Design review of the part built by this model. Coordinates are the model's own, in mm. A direction names the side the tool comes from. Coordinates: 2 decimals unless noted, no trailing zeros. Write each loop counter-clockwise with the first axis right and the second up, starting at its lowest first coordinate (ties: lowest second). Pieces come first, ordered by that corner, then holes.
Q1. For probe 1 along Y at (x, z) = (13, -22); probe 2 along Y at (x, z) = (19, -21); probe 3 along Z at (x, y) = (21, -9.25), list the stretches that pass through material, from the lowest coordinate up.
Q2. Insertion check: pin 1 (17 mm diameter, centred on x = 12, z = 0.5, fed in from -Y); pin 2 (2 mm diameter, centred on x = 22, y = -1, fed in from -Z); pin 3 (5 mm diameter, centred on y = 0, z = 21, fed in from +X); pin 4 (6.5 mm diameter, centred on y = 1.5, z = 29, fed in from -X). Each pin has a flat end and moves straight along its axis. Give the tip position at first contact, or say it passes through.
Q3. Take a section at A-A (x = 19.5). Give the boundary of the cut face in (y, z).
Q4. Take a section at C-C (y = 3). Give the boundary of the cut face in (x, z).
Q5. Take a section at B-B (x = 31). Give the boundary of the cut face in (y, z) (3 decimals).
Q6. Machinability: for faces 4 (the cylindrical face through (27.34, 11.01, -1.82)), 5 (the flat face through (10.364, 0, 27)), 6 (the flat face through (28, 6, 0)), which of the approach directions +Z, -Z, +X, -X, +Y, -Y give a long, thin tool a straight path to every point of the face, cutting with its end or side? Answer none if there is none.
Q7. Mouldability with a two-part tool opening along Y and no side actions: class faces 1 (the cylindrical face through (25.25, -8.03, -2.76)), 2 (the flat face through (24, 12, -2)), 3 (the cylindrical face through (32.84, 0.08, 4.7)) as pulls with the +Y half, pulls with the -Y half, needs draft (parallel to the pull), parting line crosses it, or undercut.
Q8. Take a section at D-D (z = 15.5). Give the boundary of the cut face in (x, y), and give its area (3 significant figures).
```python
from build123d import *

# Parameters (mm, degrees)
F0_R     = 2
F1_DEPTH = 6
F2_DEPTH = 12
F4_DEPTH = 2
F6_DEPTH = 2


with BuildPart() as f1:
    # F0 (on Front) → F1 (new body, symmetric)
    with BuildSketch(Plane.XZ):
        with BuildLine():
            Line((24.215026, 28.858344), (10.364281, 33.899603))
            Line((10.364281, 33.899603), (10.364281, 25.364181))
            ThreePointArc((10.364281, 25.364181), (27.303004, -2.303471), (5.968233, -26.742105))
            Line((5.968233, -26.742105), (5.968233, -35.4))
            Line((5.968233, -35.4), (12.884546, -35.4))
            Line((12.884546, -35.4), (32.624816, -18.835947))
            Line((32.624816, -18.835947), (37.099572, 6.541656))
            Line((37.099572, 6.541656), (24.215026, 28.858344))
        make_face()
        with Locations((10.764081, -29.574071)):
            Circle(F0_R, mode=Mode.SUBTRACT)
        with Locations((27.255351, -15.735884)):
            Circle(F0_R, mode=Mode.SUBTRACT)
        with Locations((20.229663, 24.108774)):
            Circle(F0_R, mode=Mode.SUBTRACT)
        with Locations((30.993642, 5.465015)):
            Circle(F0_R, mode=Mode.SUBTRACT)
        with BuildLine():
            ThreePointArc((5.968233, -26.742105), (27.303004, -2.303471), (10.364281, 25.364181))
            Line((10.364281, 25.364181), (10.364281, 23.189258))
            ThreePointArc((10.364281, 23.189258), (25.293606, -2.322395), (5.968233, -24.688868))
            Line((5.968233, -24.688868), (5.968233, -26.742105))
        make_face()
    extrude(amount=F1_DEPTH, both=True)

    # F0 (on Front) → F2 (join, symmetric)
    with BuildSketch(Plane.XZ):
        with BuildLine():
            ThreePointArc((5.968233, -24.688868), (25.293606, -2.322395), (10.364281, 23.189258))
            Line((10.364281, 23.189258), (10.364281, 21.189258))
            ThreePointArc((10.364281, 21.189258), (23.471393, -2.344502), (5.968233, -22.820674))
            Line((5.968233, -22.820674), (5.968233, -24.688868))
        make_face()
    extrude(amount=F2_DEPTH, both=True)

    # F3 (on face) → F4 (join)
    with BuildSketch(Plane.XZ.offset(12)):
        with BuildLine():
            Line((5.968233, -24.688868), (5.968233, -26.742105))
            ThreePointArc((5.968233, -26.742105), (27.303004, -2.303471), (10.364281, 25.364181))
            Line((10.364281, 25.364181), (10.364281, 23.189258))
            ThreePointArc((10.364281, 23.189258), (25.293606, -2.322395), (5.968233, -24.688868))
        make_face()
    extrude(amount=-F4_DEPTH)

    # F5 (on face) → F6 (join)
    with BuildSketch(Plane(origin=(0, 12, 0), x_dir=(-1, 0, 0), z_dir=(0, 1, 0))):
        with BuildLine():
            ThreePointArc((-10.364281, 25.364181), (-27.303004, -2.303471), (-5.968233, -26.742105))
            Line((-5.968233, -26.742105), (-5.968233, -24.688868))
            ThreePointArc((-5.968233, -24.688868), (-25.293606, -2.322395), (-10.364281, 23.189258))
            Line((-10.364281, 23.189258), (-10.364281, 25.364181))
        make_face()
    extrude(amount=-F6_DEPTH)


solid = f1.part
```
Response:
1. probe 1: y = -12 to -10, -6 to 6, 10 to 12
1. probe 2: y = -6 to 6
1. probe 3: z = -14.29 to -10.74, 10.74 to 14.29
2. pin 1: passes through
2. pin 2: stops at z = -28.59
2. pin 3: stops at x = 30.2
2. pin 4: stops at x = 10.36
3. outline: (-12, -19.25) - (-10, -19.25) - (-10, -16.28) - (-6, -16.28) - (-6, -29.85) - (6, -29.85) - (6, -16.28) - (10, -16.28) - (10, -19.25) - (12, -19.25) - (12, -13.27) - (-12, -13.27) - close; (-12, 13.27) - (12, 13.27) - (12, 19.25) - (10, 19.25) - (10, 16.28) - (6, 16.28) - (6, 22.25) - (-6, 22.25) - (-6, 16.28) - (-10, 16.28) - (-10, 19.25) - (-12, 19.25) - close; (-6, 25.97) - (6, 25.97) - (6, 30.57) - (-6, 30.57) - close
4. outline: (5.97, -35.4) - (12.88, -35.4) - (32.62, -18.84) - (37.1, 6.54) - (24.22, 28.86) - (10.36, 33.9) - (10.36, 21.19) arc R23.59 cw to (5.97, -22.82) - close; hole circle Ø4 at (10.76, -29.57); hole circle Ø4 at (20.23, 24.11); hole circle Ø4 at (27.26, -15.74); hole circle Ø4 at (30.99, 5.47)
5. outline: (-6, -20.199) - (6, -20.199) - (6, 3.465) - (-6, 3.465) - close; (-6, 7.465) - (6, 7.465) - (6, 17.106) - (-6, 17.106) - close
6. face 4: +X, +Y
6. face 5: +Z, -X, +Y, -Y
6. face 6: +X
7. face 1: undercut
7. face 2: pulls with the +Y half
7. face 3: needs draft
8. outline: (17.78, -12) - (22.59, -12) - (22.59, -10) - (20.12, -10) - (20.12, -6) - (31.93, -6) - (31.93, 6) - (20.12, 6) - (20.12, 10) - (22.59, 10) - (22.59, 12) - (17.78, 12) - close
8. area: 208 mm2
